from build123d import *

# Parameters (mm, degrees)
ESQUISSE1_R             = 3.985
BOSS_EXTRU_1_DEPTH      = 2
ENL_V_MAT_EXTRU_1_DEPTH = 0.3


with BuildPart() as part:
    # Esquisse1 → Boss.-Extru.1 (new body)
    with BuildSketch(Plane(origin=(0, 0, 0), x_dir=(0, 1, 0), z_dir=(0, 0, 1))):
        with BuildLine():
            ThreePointArc((-7.808836578, 1.128791965), (0, -7.89), (7.808836578, 1.128791965))
            ThreePointArc((7.808836578, 1.128791965), (5.288552874, 36.18), (7.808836578, 71.231208035))
            ThreePointArc((7.808836578, 71.231208035), (0, 80.25), (-7.808836578, 71.231208035))
            ThreePointArc((-7.808836578, 71.231208035), (-5.288552874, 36.18), (-7.808836578, 1.128791965))
        make_face()
        with Locations(Location((0, 0, 0), (0, 0, 270))):
            Circle(ESQUISSE1_R, mode=Mode.SUBTRACT)
        with Locations(Location((0, 72.36, 0), (0, 0, 270))):
            Circle(ESQUISSE1_R, mode=Mode.SUBTRACT)
    extrude(amount=BOSS_EXTRU_1_DEPTH)

    # Esquisse2 → Enlèv. mat.-Extru.1 (cut)
    with BuildSketch(Plane.XY.offset(2)):
        with BuildLine():
            Line((-64.419013619, 1.363972656), (-63.790808491, 1.363972656))
            Line((-63.790808491, 1.363972656), (-63.790808491, -0.959544972))
            add(Edge.make_bspline(
                [(-63.790808491, -0.959544972), (-63.791038809, -1.003953677), (-63.791482588, -1.089520485), (-63.795925603, -1.212705101), (-63.801933342, -1.32564701), (-63.810585066, -1.428165243), (-63.823435245, -1.520254841), (-63.837977746, -1.60214556), (-63.854022161, -1.674171081), (-63.881125115, -1.754778845), (-63.923201666, -1.844042774), (-63.986696382, -1.940460503), (-64.065767627, -2.02423108), (-64.156831583, -2.096995508), (-64.260655531, -2.154611171), (-64.374847611, -2.196255927), (-64.499042779, -2.221134792), (-64.58506355, -2.224195282), (-64.629350157, -2.225770934)],
                knots=[0, 0, 0, 0, 1.22248561, 2.355488409, 3.392943897, 4.335991845, 5.186735882, 5.951517034, 6.625683685, 7.215700098, 8.28923535, 9.333114649, 10.380102123, 11.447198135, 12.530158036, 13.633358744, 14.781567393, 16, 16, 16, 16], degree=3))
            add(Edge.make_bspline(
                [(-64.629350157, -2.225770934), (-64.675492772, -2.224342411), (-64.766504027, -2.221524808), (-64.899981406, -2.197526059), (-65.028269852, -2.159048845), (-65.150705669, -2.10341541), (-65.268966265, -2.033727017), (-65.380905318, -1.947285348), (-65.488859962, -1.846771339), (-65.552856134, -1.769639411), (-65.585680285, -1.730077825)],
                knots=[0, 0, 0, 0, 0.990984786, 1.954608977, 2.90473533, 3.862451285, 4.837525908, 5.848096122, 6.896271184, 8, 8, 8, 8], degree=3))
            Line((-65.585680285, -1.730077825), (-65.110319708, -1.290474459))
            add(Edge.make_bspline(
                [(-65.110319708, -1.290474459), (-65.085430365, -1.318617278), (-65.038855713, -1.371280057), (-64.968669084, -1.439953614), (-64.905356964, -1.495124891), (-64.845674591, -1.53492043), (-64.789353767, -1.562971842), (-64.73518271, -1.583178063), (-64.681472832, -1.594615932), (-64.645990448, -1.596597398), (-64.628649035, -1.597565805)],
                knots=[0, 0, 0, 0, 1.529509877, 2.862124173, 3.996688592, 4.944357383, 5.774364335, 6.554177287, 7.293378699, 8, 8, 8, 8], degree=3))
            add(Edge.make_bspline(
                [(-64.628649035, -1.597565805), (-64.611864478, -1.596690518), (-64.579593293, -1.595007627), (-64.535219176, -1.576300168), (-64.497808939, -1.54692867), (-64.473180247, -1.513162323), (-64.457485253, -1.478644025), (-64.447678724, -1.445276783), (-64.438372312, -1.405278504), (-64.430916222, -1.358669235), (-64.425282386, -1.30484102), (-64.422474327, -1.244447332), (-64.419059366, -1.177161813), (-64.41902941, -1.130157038), (-64.419013619, -1.105378305)],
                knots=[0, 0, 0, 0, 1.003927327, 1.930222208, 2.840933547, 3.835773585, 4.407906147, 5.114514582, 5.922289074, 6.876303333, 7.950072246, 9.174518422, 10.510537432, 12, 12, 12, 12], degree=3))
            Line((-64.419013619, -1.105378305), (-64.419013619, 1.363972656))
        make_face()
    extrude(amount=-ENL_V_MAT_EXTRU_1_DEPTH, mode=Mode.SUBTRACT)


solid = part.part
Build history of the part. All positions in model axes, mm. A direction names the side the tool comes from. Round coordinates to 2 decimals unless told otherwise and drop trailing zeros. Loops run counter-clockwise (first coordinate to the right, second up) from the corner with the lowest first, then second, coordinate; pieces in that order, holes last. Notation, with made-up numbers: (-30, 63) -> (22, 63) arc R15 cw to (22, 85) -> close; hole circle Ø4 at (33.25, 45). An arc over 180 degrees is marked (long way). Answer in a Markdown table with one row per item.
Item 1: Mould opens along X. For faces 3 (the flat face through (-37, 0, 0)), 4 (the cylindrical face through (-0.86, -3.89, 0.99)), 5 (the cylindrical face through (-76.34, 0.18, 0.99)) say: +X half, -X half, draft (parallel to the pull), parting line (faces both ways), or undercut.
Answers below:
| item | result |
|---|---|
| face 3 | draft |
| face 4 | undercut |
| face 5 | undercut |
Item 2: Saw through at A-A (y = 0). Write the cut outline in (x, z) (3 decimals), and give its area (3 significant figures).
Answers below:
| item | result |
|---|---|
| outline | (-80.25, 0) -> (-76.345, 0) -> (-76.345, 2) -> (-80.25, 2) -> close; (-68.375, 0) -> (-3.985, 0) -> (-3.985, 2) -> (-63.791, 2) -> (-63.791, 1.7) -> (-64.419, 1.7) -> (-64.419, 2) -> (-68.375, 2) -> close; (3.985, 0) -> (7.89, 0) -> (7.89, 2) -> (3.985, 2) -> close |
| area | 144 mm² |
Item 3: Drill centre lines: L1, parallel to Y at x = -72.36, z = 0.7 (3 decimals); L2, parallel to X at y = -2, z = 1.6; L3, parallel to X at y = 2.75, z = 1.9. Where is each one in solid material? Low to high. Write a range as [from, to].
Answers below:
| item | result |
|---|---|
| L1 | y = [-7.89, -3.985], [3.985, 7.89] |
| L2 | x = [-79.99, -75.81], [-68.91, -3.45], [3.45, 7.63] |
| L3 | x = [-79.76, -75.24], [-69.48, -2.88], [2.88, 7.4] |
Item 4: Saw through at C-C (z = 1.2). Write the cut outline in (x, y) (3 decimals).
Answers below:
| item | result |
|---|---|
| outline | (-71.231, -7.809) arc R245 cw to (-1.129, -7.809) arc R7.89 ccw (long way) to (-1.129, 7.809) arc R245 cw to (-71.231, 7.809) arc R7.89 ccw (long way) to start; hole circle Ø7.97 at (-72.36, 0); hole circle Ø7.97 at (0, 0) |
Item 5: Saw through at D-D (y = -6.5). Write the cut outline in (x, z), and give its area (3 significant figures).
Answers below:
| item | result |
|---|---|
| outline | (-76.83, 0) -> (-60.51, 0) -> (-60.51, 2) -> (-76.83, 2) -> close; (-11.85, 0) -> (4.47, 0) -> (4.47, 2) -> (-11.85, 2) -> close |
| area | 65.3 mm² |
Item 6: Saw through at B-B (x = 0). Write the cut outline in (y, z) (3 decimals).
Answers below:
| item | result |
|---|---|
| outline | (-7.89, 0) -> (-3.985, 0) -> (-3.985, 2) -> (-7.89, 2) -> close; (3.985, 0) -> (7.89, 0) -> (7.89, 2) -> (3.985, 2) -> close |
Item 7: Which spindle directions (+Z, -Z, +X, -X, +Y, -Y) get a long thin tool onto all of the face, cutting with end or side? Do faces 1 (the cylindrical face through (-35.69, 5.29, 0.99)), 2 (the flat face through (-64, -1, 1.7)). Say none if no direction does.
Answers below:
| item | result |
|---|---|
| face 1 | +Z, -Z, +Y |
| face 2 | +Z |
